```python
from build123d import *

# Parameters (mm, degrees)
SKETCH_1_W          = 18
SKETCH_1_H          = 120
EXTRUDE_1_DEPTH     = 5
SKETCH_2_R          = 3.25
CUT_EXTRUDE_1_DEPTH = 30
FILLET_1_R          = 8


with BuildPart() as part:
    # 스케치1 → 보스-돌출1 (new body)
    with BuildSketch(Plane.XY):
        with Locations((-0.193251534, 50.955788216)):
            Rectangle(SKETCH_1_W, SKETCH_1_H)
    extrude(amount=EXTRUDE_1_DEPTH)

    # 스케치2 → 컷-돌출1 (cut)
    with BuildSketch(Plane.XY.offset(5)):
        with Locations((0, 100.955788216)):
            Circle(SKETCH_2_R)
        with Locations((0, 0.955788216)):
            Circle(SKETCH_2_R)
    extrude(amount=-CUT_EXTRUDE_1_DEPTH, mode=Mode.SUBTRACT)

    # 필렛1
    fillet_1_edges = [part.edges().sort_by_distance(p)[0] for p in [
        (-9.193251534, 110.955788216, 2.5),
        (-9.193251534, -9.044211784, 2.5),
        (8.806748466, -9.044211784, 2.5),
        (8.806748466, 110.955788216, 2.5),
    ]]
    fillet(fillet_1_edges, radius=FILLET_1_R)


solid = part.part
```
Can you work these out from the model? Positions are in its coordinate system, mm. Give positions to 0.01 mm unless a question says otherwise; leave off trailing zeros. Loops run counter-clockwise (first coordinate to the right, second up) from the corner with the lowest first, then second, coordinate; pieces in that order, holes last. Notation, with made-up numbers: M 74,-29.5 L 109,-29.5 A22 ccw 109,-12.5 Z; hole C 63.5,34 d9. An arc over 180 degrees is marked long. One line per question, with ' | ' between items. Start each with the question number.
Q1. If we mould it in two halves opening along X, with no side actions, what happens to faces 1 (the flat face through (0, 52, 0)), 2 (the cylindrical face through (6.401, -6.763, 2.535)), 3 (the cylindrical face through (-0.705, 97.783, 2.535))? For each: +X half, -X half, draft (parallel to the pull), parting line (faces both ways), or undercut.
Q2. For pin 1 Ø3 at (x, z) = (7, 3) entering from +Y; pin 2 Ø1.5 at (x, z) = (6, 1) entering from +Y; pin 3 Ø6 at (x, y) = (0, 100.96) entering from -Z, each with a flat end and sliding along its axis, tell me the tip position at first contact or that it passes through.
Q3. If we section it at B-B (x = -7.5): Please give me the cut outline in (y, z), plus the area to 3 significant figures.
Q4. If we section it at A-A (z = 0.95): Please give me the cut outline in (x, y), plus the area to 3 significant figures.
Q5. If I drill on line 1 (Y direction, x = 0, z = 3.55); line 2 (Y direction, x = 2.25, z = 3.2); line 3 (X direction, y = 102.5, z = 0.35), over which ranges is the centre line in solid material (lowest first)? Write a range as from..to.
Computed:
1) face 1: draft | face 2: +X half | face 3: undercut
2) pin 1: stops at y = 109.43 | pin 2: stops at y = 109.61 | pin 3: passes through
3) outline: M -5.97,0 L 107.88,0 L 107.88,5 L -5.97,5 Z | area: 569 mm²
4) outline: M -9.19,-1.04 A8 ccw -1.19,-9.04 L 0.81,-9.04 A8 ccw 8.81,-1.04 L 8.81,102.96 A8 ccw 0.81,110.96 L -1.19,110.96 A8 ccw -9.19,102.96 Z; hole C 0,0.96 d6.5; hole C 0,100.96 d6.5 | area: 2,040 mm²
5) line 1: y = -9.04..-2.29, 4.21..97.71, 104.21..110.96 | line 2: y = -8.91..-1.39, 3.3..98.61, 103.3..110.82 | line 3: x = -9.19..-2.86, 2.86..8.81
